Geometry: final body of the model. Coordinates: model frame, mm. A direction names the side the tool comes from. Round coordinates to 2 decimals unless told otherwise and drop trailing zeros. Return JSON: item names as keys, results as strings.
Autodesk Inventor part; units mm, degrees
ref_plane "YZ Plane" through (0, 0, 0) normal (1, 0, 0) x (0, 1, 0)
ref_plane "XZ Plane" through (0, 0, 0) normal (0, 1, 0) x (-1, 0, 0)
ref_plane "XY Plane" through (0, 0, 0) normal (0, 0, 1) x (1, 0, 0)
sketch "Sketch1" plane through (0, 0, 0) normal (0, 1, 0) x (-1, 0, 0)
  line L0 (0, 0) -> (0, -150)
  line L1 (0, -150) -> (50, -150)
  line L2 (0, 0) -> (50, -44.9152) construction
  line L3 (50, -44.9152) -> (50, -150) construction
  spline S0 degree 2 poles (0, 0) (50, -44.9152) (50, -150) knots 1 1 1 2 2 2
  dimension "d0" = 150
  dimension "d2" = 50
extrude "Extrusion7" add sketch "Sketch1" along normal blind 150
sketch "Sketch5" plane through (0, 0, -150) normal (0, 0, -1) x (-1, 0, 0)
  line L0 (0, 0) -> (0, 150)
  line L1 (0, 0) -> (20, 0)
  line L2 (0, 0) -> (50, 0)
  line L3 (20, 0) -> (20, 75)
  line L4 (25.15, 80.15) -> (14.85, 80.15)
  line L5 (14.85, 80.15) -> (14.85, 69.85)
  line L6 (14.85, 69.85) -> (25.15, 69.85)
  line L7 (25.15, 69.85) -> (25.15, 80.15)
  line L8 (25.15, 80.15) -> (14.85, 69.85) construction
  line L9 (14.85, 80.15) -> (25.15, 69.85) construction
  dimension "d57" = 20
  dimension "d58" = 75
  dimension "d59" = 10.3
  dimension "d60" = 10.3
extrude "Extrusion8" cut sketch "Sketch5" against normal blind 10
sketch "Sketch6" plane through (0, 0, 0) normal (0, -1, 0) x (1, 0, 0)
  line L0 (0, 0) -> (0, -150)
  line L1 (0, -150) -> (-20, -150)
  line L2 (0, -150) -> (-50, -150)
  line L3 (-20, -150) -> (-20, -100)
  line L4 (-25.15, -105.15) -> (-14.85, -105.15)
  line L5 (-14.85, -105.15) -> (-14.85, -94.85)
  line L6 (-14.85, -94.85) -> (-25.15, -94.85)
  line L7 (-25.15, -94.85) -> (-25.15, -105.15)
  line L8 (-25.15, -105.15) -> (-14.85, -94.85) construction
  line L9 (-14.85, -105.15) -> (-25.15, -94.85) construction
  dimension "d51" = 20
  dimension "d52" = 50
  dimension "d53" = 10.3
  dimension "d54" = 10.3
extrude "Extrusion9" cut sketch "Sketch6" against normal blind 10
sketch "Sketch7" plane through (0, 150, 0) normal (0, 1, 0) x (1, 0, 0)
  line L0 (0, 150) -> (-50, 150)
  line L1 (0, 150) -> (-20, 150)
  line L2 (-20, 150) -> (-20, 100)
  line L3 (-15, 95) -> (-25, 95)
  line L4 (-25, 95) -> (-25, 105)
  line L5 (-25, 105) -> (-15, 105)
  line L6 (-15, 105) -> (-15, 95)
  line L7 (-15, 95) -> (-25, 105) construction
  line L8 (-25, 95) -> (-15, 105) construction
  point P0 (0, 0)
  dimension "d61" = 20
  dimension "d62" = 50
  dimension "d63" = 10
  dimension "d64" = 10
extrude "Extrusion10" add sketch "Sketch7" along normal blind 10
sketch "Sketch8" plane through (0, 0, 0) normal (1, 0, 0) x (0, 0, -1)
  line L0 (0, 0) -> (0, 150)
  line L1 (0, 75) -> (75, 75) construction
  line L2 (0, 150) -> (150, 150)
  circle A0 centre (75, 75) radius 6.25
  line L3 (75, 75) -> (86, 75)
  line L4 (75, 75) -> (80.5, 84.5263)
  line L5 (75, 75) -> (69.5, 84.5263)
  line L6 (75, 75) -> (64, 75)
  line L7 (75, 75) -> (69.5, 65.4737)
  line L8 (75, 75) -> (80.5, 65.4737)
  line L9 (80.5, 65.4737) -> (86, 75)
  line L10 (80.5, 84.5263) -> (86, 75)
  line L11 (69.5, 84.5263) -> (80.5, 84.5263)
  line L12 (69.5, 84.5263) -> (64, 75)
  line L13 (64, 75) -> (69.5, 65.4737)
  line L14 (80.5, 65.4737) -> (69.5, 65.4737)
  dimension "d67" = 75
  dimension "d69" = 12.5
  dimension "d70" = 11
  dimension "d73" = 360
extrude "Extrusion11" cut sketch "Sketch8" against normal blind 100
extrude "Extrusion12" add sketch "Sketch8" against normal blind 5 contours L3 L9 L8 A0 | A0 L4 L10 L3 | A0 L5 L11 L4 | L8 L14 L7 A0 | A0 L6 L12 L5 | L7 L13 L6 A0
properties part number "3DPrintShapeCorner"
Q1. Reachability of faces 4 (the flat face through (-24.38, 79.83, -83.21)), 5 (the flat face through (-20, 155, -105)), 6 (the flat face through (-20, 69.85, -145)), 7 (the flat face through (-25.15, 5, -100)) from +Z, -Z, +X, -X, +Y, -Y: full face, straight path, thin tool, end or side. Return the list, or none.
Determined:
{"face 4": "-X", "face 5": "-Z, +X, -X, +Y", "face 6": "-Z", "face 7": "-Y"}
Q2. Material intervals for L1, parallel to Y at x = -1, z = -75; L2, parallel to Y at x = -39.5, z = -95; L3, parallel to Z at x = -3.65, y = 75, sorted ascending.
Determined:
{"L1": "y = 0 to 68.75, 81.25 to 150", "L2": "y = 0 to 150", "L3": "z = -150 to -81.25, -68.75 to -3.42"}
Q3. Pin query (flat end, axial travel): pin 1 (3 mm diameter, centred on x = -22, y = 74.5, fed in from -Z); pin 2 (5 mm diameter, centred on x = -19, z = -90.5, fed in from +Y); pin 3 (3 mm diameter, centred on y = 153.5, z = -99, fed in from +X). Return the tip coordinate at first contact, or that it passes through.
Determined:
{"pin 1": "stops at z = -140", "pin 2": "stops at y = 150", "pin 3": "stops at x = -15"}
Q4. Pull-direction query (Z, two-part tool) for faces 1 (the flat face through (-24, 84.526, -75)), 2 (the flat face through (-14.85, 75, -145)), 3 (the flat face through (-20, 75, -140)); classes: pulls with the +Z half, pulls with the -Z half, needs draft (parallel to the pull), parting line crosses it, or undercut.
Determined:
{"face 1": "undercut", "face 2": "needs draft", "face 3": "pulls with the -Z half"}
